Source: CAD feature listing. Evaluate the final solid. Frame: model axes, mm. Face numbers are marked on the shaded views. A direction names the side the tool comes from. Coordinates: 2 decimals unless noted, no trailing zeros. Order: outer loops, then holes, each group sorted by start corner. A loop starts at its lowest first (then second) coordinate and runs counter-clockwise, first axis right, second up. Notation, with made-up numbers: (-11.75, -26.5) -> (45.25, -26.5) arc R16 ccw to (45.25, 2.5) -> close; hole circle Ø9 at (87.25, -17.75). An arc over 180 degrees is marked (long way). Put each result on its own line as item: value.
from build123d import *

# Parameters (mm, degrees)
EXTRUDE_2_DEPTH          = 12.2
SKETCH_5_W               = 1.5
SKETCH_5_H               = 8.35
CUT_EXTRUDE_1_DEPTH      = 22.5
SKETCH_6_R               = 1.4
EXTRUDE_3_DEPTH          = 2.5
SKETCH_7_W               = 12.2
SKETCH_7_H               = 1
CUT_EXTRUDE_2_DEPTH      = 1
CUT_EXTRUDE_2_DEPTH_BACK = 32.1


with BuildPart() as part:
    # 草图4 → 凸台-拉伸2 (new body)
    with BuildSketch(Plane.XY):
        Polygon((-11.55, 0), (11.55, 0), (11.55, 17), (16.05, 17), (16.05, -4.5), (-16.05, -4.5), (-16.05, 17), (-11.55, 17), align=None)
    extrude(amount=EXTRUDE_2_DEPTH)

    # 草图5 → 切除-拉伸1 (cut, through all)
    with BuildSketch(Plane.XZ.offset(4.5)):
        with Locations((-10.8, 4.175)):
            Rectangle(SKETCH_5_W, SKETCH_5_H)
    extrude(amount=-CUT_EXTRUDE_1_DEPTH, mode=Mode.SUBTRACT)

    # 草图6 → 凸台-拉伸3 (add)
    with BuildSketch(Plane(origin=(0, 17, 0), x_dir=(1, 0, 0), z_dir=(0, 1, 0))):
        with Locations((13.8, -6.1)):
            Circle(SKETCH_6_R)
        with Locations((-13.8, -6.1)):
            Circle(SKETCH_6_R)
    extrude(amount=EXTRUDE_3_DEPTH)

    # 草图7 → 切除-拉伸2 (cut, two sides)
    with BuildSketch(Plane(origin=(16.05, 0, 0), x_dir=(0, 0, -1), z_dir=(1, 0, 0))) as cut_extrude_2_sk:
        with Locations((-6.1, -4)):
            Rectangle(SKETCH_7_W, SKETCH_7_H)
    extrude(amount=CUT_EXTRUDE_2_DEPTH, mode=Mode.SUBTRACT)
    extrude(cut_extrude_2_sk.sketch, amount=-CUT_EXTRUDE_2_DEPTH_BACK, mode=Mode.SUBTRACT)


solid = part.part
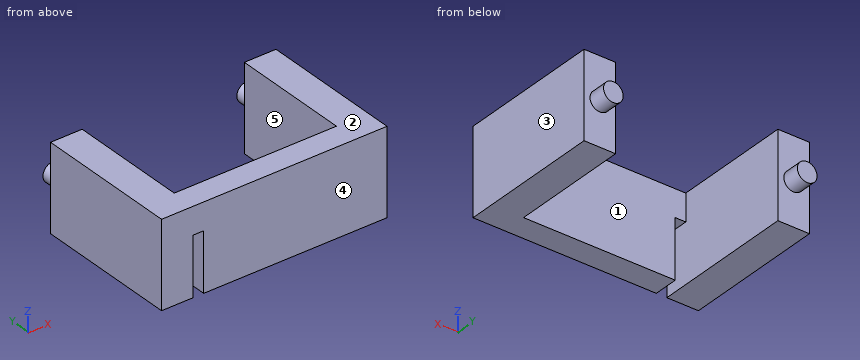
1. Cut plane A-A on z = 6.1. Output: boundary loops of the cut face in (x, y), plus the area to 3 significant figures.
Numbers:
outline: (-16.05, -3.5) -> (-11.55, -3.5) -> (-11.55, 17) -> (-12.4, 17) -> (-12.4, 19.5) -> (-15.2, 19.5) -> (-15.2, 17) -> (-16.05, 17) -> close; (-10.05, -3.5) -> (16.05, -3.5) -> (16.05, 17) -> (15.2, 17) -> (15.2, 19.5) -> (12.4, 19.5) -> (12.4, 17) -> (11.55, 17) -> (11.55, 0) -> (-10.05, 0) -> close
area: 274 mm2
2. First-contact query: pin 1 (6 mm diameter, centred on x = 2, z = 6.5, fed in from +Y); pin 2 (1.3 mm diameter, centred on x = 13, z = 4, fed in from +Y). Flat tips, straight axial feed; report the tip coordinate or a pass-through.
Numbers:
pin 1: stops at y = 0
pin 2: stops at y = 17
3. Ray query, line 1 along X through (y, z) = (11.25, 1); line 2 along Y through (x, z) = (8.5, 6.75); line 3 along Y through (x, z) = (13, 8.75). Return the intervals inside material, ascending.
Numbers:
line 1: x = -16.05 to -11.55, 11.55 to 16.05
line 2: y = -3.5 to 0
line 3: y = -3.5 to 17
4. Pull-direction query (X, two-part tool) for the marked faces 3, 4 and 5; classes: pulls with the +X half, pulls with the -X half, needs draft (parallel to the pull), parting line crosses it, or undercut.
Numbers:
face 3: pulls with the +X half
face 4: needs draft
face 5: undercut
5. Cut plane C-C on x = -13.8. Output: boundary loops of the cut face in (y, z).
Numbers:
outline: (-3.5, 0) -> (17, 0) -> (17, 4.7) -> (19.5, 4.7) -> (19.5, 7.5) -> (17, 7.5) -> (17, 12.2) -> (-3.5, 12.2) -> close
6. Cut plane B-B on y = 5. Output: boundary loops of the cut face in (x, z).
Numbers:
outline: (-16.05, 0) -> (-11.55, 0) -> (-11.55, 12.2) -> (-16.05, 12.2) -> close; (11.55, 0) -> (16.05, 0) -> (16.05, 12.2) -> (11.55, 12.2) -> close
7. Cut plane D-D on z = 9.25. Output: boundary loops of the cut face in (x, y).
Numbers:
outline: (-16.05, -3.5) -> (16.05, -3.5) -> (16.05, 17) -> (11.55, 17) -> (11.55, 0) -> (-11.55, 0) -> (-11.55, 17) -> (-16.05, 17) -> close
8. Set-up query: the marked faces 1 and 2. Return all of +Z, -Z, +X, -X, +Y, -Y with unobstructed straight access to the full face (end or side cutting, diameter ignored); none if empty.
Numbers:
face 1: +Z, -Z, +Y
face 2: +Z, +X, -X, +Y, -Y
